Geometry: final body of the model. Coordinates: model frame, mm. A direction names the side the tool comes from. Coordinates: 2 decimals unless noted, no trailing zeros. Order: outer loops, then holes, each group sorted by start corner. A loop starts at its lowest first (then second) coordinate and runs counter-clockwise, first axis right, second up. Notation, with made-up numbers: (74.25, 8) -> (104.25, 8) arc R6 cw to (104.25, 18) -> close; hole circle Ø8 at (31.5, -9.75). An arc over 180 degrees is marked (long way). Answer in a Markdown table with one row per item. Add a question column.
1) Section query C-C on y = 27. Return the cut outline in (x, z).
2) Contact query for a flat-ended pin moving along its axis: P1, Ø12, axis at x = 269, z = 233.5, coming from the -Y side. Output: stop coordinate, or through.
3) Set-up query: faces 4 (the face through (-7, 25, 300)), 5 (the face through (400, 20, 3)). Return all of +Z, -Z, +X, -X, +Y, -Y with unobstructed straight access to the full face (end or side cutting, diameter ignored); none if empty.
4) Ray query, line 1 (X direction, y = 35, z = 87); line 2 (Z direction, x = 97.5, y = 20); line 3 (Z direction, x = 193, y = 43). Return the intervals inside material, ascending. Write a range as from..to.
5) Pull-direction query (Z, two-part tool) for faces 1 (the face through (-7, 25, -300)), 2 (the face through (-35, 40, 212)), 3 (the face through (-7, 0, -204)); classes: +Z half, -Z half, draft (parallel to the pull), parting line (faces both ways), or undercut.
6) Section query A-A on z = 52. Return the cut outline in (x, y), then the cut area to 3 significant figures.
7) Section query B-B on x = -0.5. Return the cut outline in (y, z).
```python
from build123d import *

# Parameters (mm, degrees)
SKETCH1_W           = 1000
SKETCH1_H           = 600
BOSS_EXTRUDE1_DEPTH = 50
SKETCH2_W           = 800
SKETCH2_H           = 400
CUT_EXTRUDE1_DEPTH  = 51
SKETCH3_W           = 880
SKETCH3_H           = 480
CUT_EXTRUDE2_DEPTH  = 10


with BuildPart() as part:
    # Sketch1 → Boss-Extrude1 (new body)
    with BuildSketch(Plane(origin=(0, 0, 0), x_dir=(1, 0, 0), z_dir=(0, 1, 0))):
        Rectangle(SKETCH1_W, SKETCH1_H)
    extrude(amount=BOSS_EXTRUDE1_DEPTH)

    # Sketch2 → Cut-Extrude1 (cut, through all)
    with BuildSketch(Plane(origin=(0, 50, 0), x_dir=(1, 0, 0), z_dir=(0, 1, 0))):
        Rectangle(SKETCH2_W, SKETCH2_H)
    extrude(amount=-CUT_EXTRUDE1_DEPTH, mode=Mode.SUBTRACT)

    # Sketch3 → Cut-Extrude2 (cut)
    with BuildSketch(Plane(origin=(0, 50, 0), x_dir=(1, 0, 0), z_dir=(0, 1, 0))):
        Rectangle(SKETCH3_W, SKETCH3_H)
    extrude(amount=-CUT_EXTRUDE2_DEPTH, mode=Mode.SUBTRACT)


solid = part.part
```
Result:
| question | item | result |
|---|---|---|
| 1 | outline | (-500, -300) -> (500, -300) -> (500, 300) -> (-500, 300) -> close; hole (-400, -200) -> (400, -200) -> (400, 200) -> (-400, 200) -> close |
| 2 | P1 | y = 0 |
| 3 | face 4 | +Z, +X, -X, +Y, -Y |
| 3 | face 5 | +Y, -Y |
| 4 | line 1 | -500..-400, 400..500 |
| 4 | line 2 | -300..-200, 200..300 |
| 4 | line 3 | -300..-240, 240..300 |
| 5 | face 1 | -Z half |
| 5 | face 2 | undercut |
| 5 | face 3 | draft |
| 6 | outline | (-500, 0) -> (-400, 0) -> (-400, 40) -> (-440, 40) -> (-440, 50) -> (-500, 50) -> close; (400, 0) -> (500, 0) -> (500, 50) -> (440, 50) -> (440, 40) -> (400, 40) -> close |
| 6 | area | 9,200 mm2 |
| 7 | outline | (0, -300) -> (50, -300) -> (50, -240) -> (40, -240) -> (40, -200) -> (0, -200) -> close; (0, 200) -> (40, 200) -> (40, 240) -> (50, 240) -> (50, 300) -> (0, 300) -> close |
